Model file for the job. Use its own axes, mm. Give positions to 0.01 mm unless a question says otherwise; leave off trailing zeros. Order: outer loops, then holes, each group sorted by start corner. A loop starts at its lowest first (then second) coordinate and runs counter-clockwise, first axis right, second up. Notation, with made-up numbers: (7, 84.5) - (61, 84.5) arc R23 cw to (61, 115.5) - close; hole circle Ø1 at (51, 70.25). An arc over 180 degrees is marked (long way). Return JSON: item names as keys, results as strings. Group by question number.
from build123d import *

# Parameters (mm, degrees)
F0_R     = 5.8656239377
F1_DEPTH = 37.5
F2_T     = -2.5
F3_R     = 2.5
F4_R     = 1


with BuildPart() as f1:
    # F0 (on Top) → F1 (new body)
    with BuildSketch(Plane.XY):
        Circle(F0_R)
    extrude(amount=F1_DEPTH)

    # F2
    f2_openings = [f1.faces().sort_by_distance(p)[0] for p in [
        (0, 0, 37.5),
    ]]
    offset(amount=F2_T, openings=f2_openings)

    # F3
    f3_edges = [f1.edges().sort_by_distance(p)[0] for p in [
        (-5.865624, 0, 0),
    ]]
    fillet(f3_edges, radius=F3_R)

    # F4
    f4_edges = [f1.edges().sort_by_distance(p)[0] for p in [
        (-5.865624, 0, 37.5),
        (-3.365624, 0, 37.5),
    ]]
    fillet(f4_edges, radius=F4_R)


solid = f1.part
(1) Slice it at A-A (y = 0). Give the cut face in (x, z).
(2) Drop flat-ended pins along their axis: pin 1 Ø1.5 at (x, y) = (1, 3) entering from +Z; pin 2 Ø5.5 at (x, y) = (-0.5, 0) entering from +Z; pin 3 Ø1.5 at (x, z) = (4.5, 18.5) entering from +Y. Give the stop position or say it passes through.
(3) Pull direction X, two halves, no side cores. Call faces 1 (the face through (5.595, 1.762, 19.262)), 2 (the face through (0, 0, 0)), 3 (the face through (0, 0, 2.5)): released by +X, released by -X, zero draft, split by the parting line, or undercut.
(4) Slice it at C-C (z = 21). Give the cut face in (x, y), and give its area (3 significant figures).
(5) Drill centre lines: L1, parallel to Y at x = 0, z = 21; L2, parallel to Z at x = -3, y = 1.25; L3, parallel to X at y = 2, z = 17. Where is each one in solid material? Low to high.
Result set:
{
 "1": {"outline": "(-5.87, 2.5) arc R2.5 ccw to (-3.37, 0) - (3.37, 0) arc R2.5 ccw to (5.87, 2.5) - (5.87, 36.5) arc R1 ccw to (4.87, 37.5) - (4.37, 37.5) arc R1 ccw to (3.37, 36.5) - (3.37, 2.5) - (-3.37, 2.5) - (-3.37, 36.5) arc R1 ccw to (-4.37, 37.5) - (-4.87, 37.5) arc R1 ccw to (-5.87, 36.5) - close"},
 "2": {"pin 1": "stops at z = 37.39", "pin 2": "stops at z = 2.5", "pin 3": "stops at y = 4.51"},
 "3": {"face 1": "split by the parting line", "face 2": "zero draft", "face 3": "undercut"},
 "4": {"outline": "circle Ø11.73 at (0, 0); hole circle Ø6.73 at (0, 0)", "area": "72.5 mm²"},
 "5": {"L1": "y = -5.87 to -3.37, 3.37 to 5.87", "L2": "z = 0 to 2.5", "L3": "x = -5.51 to -2.71, 2.71 to 5.51"}
}
